from build123d import *

# Parameters (mm, degrees)
BOSS_EXTRUDE1_DEPTH = 2
CUT_EXTRUDE1_DEPTH  = 3


with BuildPart() as part:
    # Sketch1 → Boss-Extrude1 (new body)
    with BuildSketch(Plane(origin=(0, 0, 0), x_dir=(1, 0, 0), z_dir=(0, 1, 0))):
        Polygon((0, 0), (3.3, 0), (3.3, 31), (2.3, 31), (2.3, 64), (33.65, 64), (33.65, 115), (-30.35, 115), (-30.35, 64), (1, 64), (1, 31), (0, 31), align=None)
    extrude(amount=BOSS_EXTRUDE1_DEPTH)

    # Sketch2 → Cut-Extrude1 (cut, through all)
    with BuildSketch(Plane(origin=(0, 2, 0), x_dir=(1, 0, 0), z_dir=(0, 1, 0))):
        Polygon((21.744274217, 105.199367621), (22.359935692, 104.411356867), (-17.828612742, 73.012621626), (-19.059935692, 74.588643133), (21.128612742, 105.987378374), align=None)
    extrude(amount=-CUT_EXTRUDE1_DEPTH, mode=Mode.SUBTRACT)


solid = part.part
Model file for the job. Use its own axes, mm. A direction names the side the tool comes from. Give positions to 0.01 mm unless a question says otherwise; leave off trailing zeros. Order: outer loops, then holes, each group sorted by start corner. A loop starts at its lowest first (then second) coordinate and runs counter-clockwise, first axis right, second up. Notation, with made-up numbers: (53.5, -34) - (105.5, -34) arc R28 cw to (105.5, -8) - close; hole circle Ø4 at (-10.5, -5). An arc over 180 degrees is marked (long way). One line per item, written item: value.
Item 1: Pin check, flat tips, straight feed: pin 1 Ø0.6 at (y, z) = (1, -13.5) entering from +X; pin 2 Ø1 at (y, z) = (1.5, -56) entering from -X; pin 3 Ø1 at (x, y) = (-20.5, 1) entering from +Z. Stop position of each tip, or through.
Response values:
pin 1: x = 3.3
pin 2: x = 1
pin 3: z = -64
Item 2: Slice it at A-A (z = -89). List the corners of the cut face in (x, y), then the cut area to 3 significant figures.
Response values:
outline: (-30.35, 0) - (-0.61, 0) - (-0.61, 2) - (-30.35, 2) - close; (2.63, 0) - (33.65, 0) - (33.65, 2) - (2.63, 2) - close
area: 122 mm2
Item 3: Slice it at B-B (x = -10). List the corners of the cut face in (y, z), then the cut area to 3 significant figures.
Response values:
outline: (0, -115) - (2, -115) - (2, -81.67) - (0, -81.67) - close; (0, -79.13) - (2, -79.13) - (2, -64) - (0, -64) - close
area: 96.9 mm2
Item 4: Tool access for faces 1 (the flat face through (33.65, 1, -89)), 2 (the flat face through (1, 1, -48)), 3 (the flat face through (3.3, 1, -15)), 4 (the flat face through (0, 1, -16)), 5 (the flat face through (0.753, 1.014, -90.068)): list every direction of +Z, -Z, +X, -X, +Y, -Y with a clear straight run to the whole face (end or side of a thin tool).
Response values:
face 1: +Z, -Z, +X, +Y, -Y
face 2: -X, +Y, -Y
face 3: +Z, +X, +Y, -Y
face 4: +Z, -X, +Y, -Y
face 5: +Y, -Y
Item 5: Slice it at D-D (z = -34). List the corners of the cut face in (x, y).
Response values:
outline: (1, 0) - (2.3, 0) - (2.3, 2) - (1, 2) - close
Item 6: Slice it at C-C (y = 1). List the corners of the cut face in (x, z).
Response values:
outline: (-30.35, -115) - (33.65, -115) - (33.65, -64) - (2.3, -64) - (2.3, -31) - (3.3, -31) - (3.3, 0) - (0, 0) - (0, -31) - (1, -31) - (1, -64) - (-30.35, -64) - close; hole (-19.06, -74.59) - (21.13, -105.99) - (22.36, -104.41) - (-17.83, -73.01) - close
Item 7: Two-plate mould, pull along Z, no slides. Class faces 6 (the flat face through (1, 0, -84)), 7 (the flat face through (2.3, 1, -47)), 8 (the flat face through (2, 1, -115)): released by +Z, released by -Z, zero draft, split by the parting line, or undercut.
Response values:
face 6: zero draft
face 7: undercut
face 8: released by -Z
Item 8: Wall check: line 1 (X direction, y = 1.5, z = -23); line 2 (X direction, y = 1.25, z = -49); line 3 (Z direction, x = -6, y = 0.55). Give the ranges that are in metal, low to high.
Response values:
line 1: 0 to 3.3
line 2: 1 to 2.3
line 3: -115 to -84.79, -82.25 to -64
